Geometry check sheet. Reference: the model listing, model coordinates, mm. A direction names the side the tool comes from. Round coordinates to 2 decimals unless told otherwise and drop trailing zeros. Loops run counter-clockwise (first coordinate to the right, second up) from the corner with the lowest first, then second, coordinate; pieces in that order, holes last.
```python
from build123d import *

# Parameters (mm, degrees)
SKETCH1_W           = 1066.8
SKETCH1_H           = 736.6
BOSS_EXTRUDE1_DEPTH = 152.4
SHELL1_T            = -6.35
SKETCH2_R           = 5.08
CUT_EXTRUDE1_DEPTH  = 7.35
SKETCH3_W           = 203.2
SKETCH3_H           = 6.35
CUT_EXTRUDE3_DEPTH  = 737.6
SKETCH4_W           = 203.2
SKETCH4_H           = 6.35
CUT_EXTRUDE4_DEPTH  = 1067.8
SKETCH6_R           = 3.175
BOSS_EXTRUDE3_DEPTH = 63.5


with BuildPart() as part:
    # Sketch1 → Boss-Extrude1 (new body)
    with BuildSketch(Plane(origin=(0, 0, 0), x_dir=(1, 0, 0), z_dir=(0, 1, 0))):
        Rectangle(SKETCH1_W, SKETCH1_H)
    extrude(amount=BOSS_EXTRUDE1_DEPTH)

    # Shell1
    shell1_openings = [part.faces().sort_by_distance(p)[0] for p in [
        (0, 152.4, 0),
    ]]
    offset(amount=SHELL1_T, openings=shell1_openings, kind=Kind.INTERSECTION)

    # Sketch2 → Cut-Extrude1 (cut, through all)
    with BuildSketch(Plane(origin=(0, 6.35, 0), x_dir=(1, 0, 0), z_dir=(0, 1, 0))):
        with Locations((-514.35, -6.35)):
            Circle(SKETCH2_R)
        with Locations((514.35, -6.35)):
            Circle(SKETCH2_R)
    extrude(amount=-CUT_EXTRUDE1_DEPTH, mode=Mode.SUBTRACT)

    # Sketch3 → Cut-Extrude3 (cut, through all)
    with BuildSketch(Plane.XY.offset(368.3)):
        with Locations((-304.8, 9.525)):
            Rectangle(SKETCH3_W, SKETCH3_H)
        with Locations((304.8, 9.525)):
            Rectangle(SKETCH3_W, SKETCH3_H)
    extrude(amount=-CUT_EXTRUDE3_DEPTH, mode=Mode.SUBTRACT)

    # Sketch4 → Cut-Extrude4 (cut, through all)
    with BuildSketch(Plane.ZY.offset(533.4)):
        with Locations((-190.5, 9.525)):
            Rectangle(SKETCH4_W, SKETCH4_H)
        with Locations((190.5, 9.525)):
            Rectangle(SKETCH4_W, SKETCH4_H)
    extrude(amount=-CUT_EXTRUDE4_DEPTH, mode=Mode.SUBTRACT)

    # Sketch6 → Boss-Extrude3 (add, symmetric)
    with BuildSketch(Plane.ZY.offset(3.175)):
        with BuildLine():
            ThreePointArc((-365.06301296, 152.4), (-371.475, 158.81198704), (-377.88698704, 152.4))
            ThreePointArc((-377.88698704, 152.4), (-371.475, 145.98801296), (-365.06301296, 152.4))
        make_face()
        with Locations((-371.475, 152.4)):
            Circle(SKETCH6_R, mode=Mode.SUBTRACT)
    extrude(amount=BOSS_EXTRUDE3_DEPTH, both=True)


solid = part.part
```
1) Gauge pin test, flat ends, axial feed: pin 1 (8 mm diameter, centred on x = 366, y = 47.5, fed in from -Z); pin 2 (5 mm diameter, centred on x = -335, z = 228.5, fed in from +Y). Record the tip position at first contact, or that the pin passes through.
Report:
pin 1: stops at z = -368.3
pin 2: stops at y = 6.35
2) Sectioned sample at D-D, the plane x = -128.5. Record the cut outline in (y, z), then the cut area to 3 significant figures.
Report:
outline: (0, -368.3) - (152.4, -368.3) - (152.4, -361.95) - (6.35, -361.95) - (6.35, 361.95) - (152.4, 361.95) - (152.4, 368.3) - (0, 368.3) - close
area: 6,530 mm2
3) Mould release check, pull along X, two halves, no side actions. Record for faces 1 (the face through (-7, 75, 368.3)), 2 (the face through (-7, 6.35, -5)), 3 (the face through (533.4, 75, 5)), 4 (the face through (-7, 78, -361.95)): +X half, -X half, draft (parallel to the pull), parting line (faces both ways), or undercut.
Report:
face 1: draft
face 2: undercut
face 3: +X half
face 4: undercut
4) Sectioned sample at C-C, the plane y = 51.5. Record the cut outline in (x, z).
Report:
outline: (-533.4, -368.3) - (533.4, -368.3) - (533.4, 368.3) - (-533.4, 368.3) - close; hole (-527.05, -361.95) - (527.05, -361.95) - (527.05, 361.95) - (-527.05, 361.95) - close
5) Access from +Z, -Z, +X, -X, +Y, -Y to the whole of each face (thin tool, end or side, straight path). Record for faces 5 (the face through (-527.05, 78, 5)), 6 (the face through (-533.4, 75, 5)).
Report:
face 5: +Y
face 6: +Z, -Z, -X, +Y, -Y
6) Sectioned sample at A-A, the plane z = -225.5. Record the cut outline in (x, y), then the cut area to 3 significant figures.
Report:
outline: (-533.4, 0) - (533.4, 0) - (533.4, 6.35) - (-533.4, 6.35) - close; (-533.4, 12.7) - (-527.05, 12.7) - (-527.05, 152.4) - (-533.4, 152.4) - close; (527.05, 12.7) - (533.4, 12.7) - (533.4, 152.4) - (527.05, 152.4) - close
area: 8,550 mm2
7) Scan lines: line 1 along X through (y, z) = (1, 6); line 2 along Z through (x, y) = (514.35, 3); line 3 along Z through (x, y) = (2.5, 120.5). Record each from-to range of solid material in increasing order.
Report:
line 1: x = -533.4 to -519.42, -509.28 to 509.28, 519.42 to 533.4
line 2: z = -368.3 to 1.27, 11.43 to 368.3
line 3: z = -368.3 to -361.95, 361.95 to 368.3
8) Sectioned sample at B-B, the plane x = 352.5. Record the cut outline in (y, z), then the cut area to 3 significant figures.
Report:
outline: (0, -368.3) - (6.35, -368.3) - (6.35, 368.3) - (0, 368.3) - close; (12.7, -368.3) - (152.4, -368.3) - (152.4, -361.95) - (12.7, -361.95) - close; (12.7, 361.95) - (152.4, 361.95) - (152.4, 368.3) - (12.7, 368.3) - close
area: 6,450 mm2
